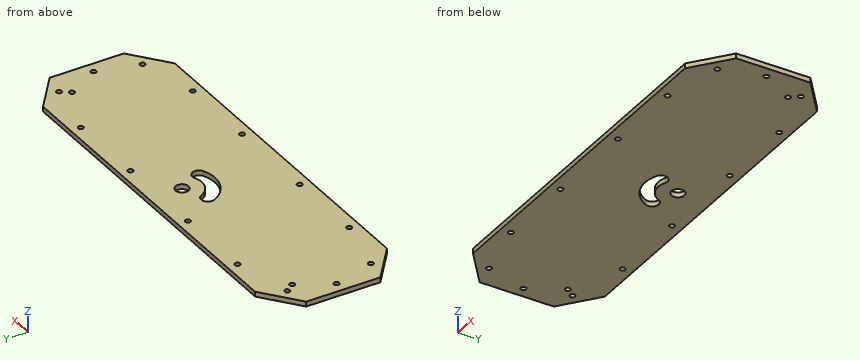
```python
from build123d import *

# Parameters (mm, degrees)
CROQUIS1_R              = 4
CROQUIS1_R_2            = 1.6
SALIENTE_EXTRUIR1_DEPTH = 3


with BuildPart() as part:
    # Croquis1 → Saliente-Extruir1 (new body)
    with BuildSketch(Plane.XY):
        Polygon((-127, 22.5), (-105, 40), (105, 40), (127, 22.5), (127, -22.5), (105, -40), (-105, -40), (-127, -22.5), align=None)
        with Locations((0, 20)):
            Circle(CROQUIS1_R, mode=Mode.SUBTRACT)
        with Locations((112.98, 25.35)):
            Circle(CROQUIS1_R_2, mode=Mode.SUBTRACT)
        with Locations((120.25, 0)):
            Circle(CROQUIS1_R_2, mode=Mode.SUBTRACT)
        with Locations((112.98, -25.35)):
            Circle(CROQUIS1_R_2, mode=Mode.SUBTRACT)
        with Locations((77.5, -33.9)):
            Circle(CROQUIS1_R_2, mode=Mode.SUBTRACT)
        with Locations((28.5, -33.9)):
            Circle(CROQUIS1_R_2, mode=Mode.SUBTRACT)
        with Locations((-28.5, -33.9)):
            Circle(CROQUIS1_R_2, mode=Mode.SUBTRACT)
        with Locations((-77.5, -33.9)):
            Circle(CROQUIS1_R_2, mode=Mode.SUBTRACT)
        with Locations((-112.98, -25.35)):
            Circle(CROQUIS1_R_2, mode=Mode.SUBTRACT)
        with Locations((-120.25, 0)):
            Circle(CROQUIS1_R_2, mode=Mode.SUBTRACT)
        with Locations((-112.98, 25.35)):
            Circle(CROQUIS1_R_2, mode=Mode.SUBTRACT)
        with Locations((-77.5, 33.9)):
            Circle(CROQUIS1_R_2, mode=Mode.SUBTRACT)
        with Locations((-28.5, 33.9)):
            Circle(CROQUIS1_R_2, mode=Mode.SUBTRACT)
        with Locations((28.5, 33.9)):
            Circle(CROQUIS1_R_2, mode=Mode.SUBTRACT)
        with Locations((77.5, 33.9)):
            Circle(CROQUIS1_R_2, mode=Mode.SUBTRACT)
        with Locations((-109, 20)):
            Circle(CROQUIS1_R_2, mode=Mode.SUBTRACT)
        with Locations((109, 20)):
            Circle(CROQUIS1_R_2, mode=Mode.SUBTRACT)
        with BuildLine():
            ThreePointArc((-18.126155741, 11.547634765), (-6.840402867, 1.206147584), (8.452365235, 1.873844259))
            ThreePointArc((8.452365235, 1.873844259), (10.387123336, 7.189548454), (5.071419141, 9.124306556))
            ThreePointArc((5.071419141, 9.124306556), (-4.10424172, 8.723688551), (-10.875693444, 14.928580859))
            ThreePointArc((-10.875693444, 14.928580859), (-16.19139764, 16.86333896), (-18.126155741, 11.547634765))
        make_face(mode=Mode.SUBTRACT)
    extrude(amount=SALIENTE_EXTRUIR1_DEPTH)


solid = part.part
```
Input: part model. Units: mm. Frame: model coordinates. Give positions to 0.01 mm unless a question says otherwise; leave off trailing zeros. Loops run counter-clockwise (first coordinate to the right, second up) from the corner with the lowest first, then second, coordinate; pieces in that order, holes last.
1) Section query B-B on y = 29.5. Return the cut outline in (x, z), and give its area (3 significant figures).
A:
outline: (-118.2, 0) - (118.2, 0) - (118.2, 3) - (-118.2, 3) - close
area: 709 mm2
2) Section query A-A on z = 0.45. Count the separate pieces of the cut face and the enclosed holes in it, and give its area (3 significant figures).
A:
separate pieces: 1
enclosed holes: 18
area: 19,100 mm2
3) Contact query for a flat-ended pin moving along its axis: pin 1 (3 mm diameter, centred on x = 120.25, y = 0, fed in from -Z). Output: stop coordinate, or through.
A:
pin 1: passes through
4) Line query: L1, parallel to Y at x = -28.5, z = 1.15; L2, parallel to X at y = 15, z = 0.3; L3, parallel to X at y = -34.5, z = 0.65. Output: solid intervals per line, ascending.
A:
L1: y = -40 to -35.5, -32.3 to 32.3, 35.5 to 40
L2: x = -127 to -18.09, -10.91 to 127
L3: x = -111.91 to -78.98, -76.02 to -29.98, -27.02 to 27.02, 29.98 to 76.02, 78.98 to 111.91
